from build123d import *

# Parameters (mm, degrees)
F0_R     = 8
F1_DEPTH = 16
F2_R     = 5.1
F3_DEPTH = 14
F4_R     = 5


with BuildPart() as f1:
    # F0 (on Top) → F1 (new body)
    with BuildSketch(Plane.XY):
        Circle(F0_R)
    extrude(amount=F1_DEPTH)

    # F2 (on face) → F3 (cut)
    with BuildSketch(Plane.XY.offset(16)):
        Circle(F2_R)
    extrude(amount=-F3_DEPTH, mode=Mode.SUBTRACT)

    # F4
    f4_edges = [f1.edges().sort_by_distance(p)[0] for p in [
        (-8, 0, 0),
    ]]
    fillet(f4_edges, radius=F4_R)


solid = f1.part
The listing builds one solid part. Answer for the finished solid, in the listing's coordinates (mm). A direction names the side the tool comes from. Round coordinates to 2 decimals unless told otherwise and drop trailing zeros. Order: outer loops, then holes, each group sorted by start corner. A loop starts at its lowest first (then second) coordinate and runs counter-clockwise, first axis right, second up. Notation, with made-up numbers: (-29.5, 83) -> (11.5, 83) arc R24 ccw to (11.5, 104) -> close; hole circle Ø1 at (0, -30.5). An arc over 180 degrees is marked (long way). Put each result on its own line as item: value.
Q1. Which of the six approach directions +Z, -Z, +X, -X, +Y, -Y give full straight-line access (tool end or side, diameter ignored) to faces 1 (the flat face through (0, 0, 0)), 2 (the flat face through (0, 0, 2))?
Results list:
face 1: -Z, +X, -X, +Y, -Y
face 2: +Z
Q2. Each of these flat-tipped pins is pushed along its axis until it touches: P1, Ø1.5, axis at x = -1, y = 1, coming from the -Z side; P2, Ø1, axis at y = -0.5, z = 2.5, coming from the -X side; P3, Ø1.5, axis at x = 3.5, z = 6.5, coming from the +Y side; P4, Ø4, axis at y = 4, z = 7.5, coming from the -X side. Where does it stop, or does it pass through?
Results list:
P1: z = 0
P2: x = -7.57
P3: y = 7.51
P4: x = -7.75
Q3. Determine the mould class of faces 3 (the flat face through (5, -2, 16)), 4 (the cylindrical face through (-1.73, -7.81, 10.42)), 5 (the cylindrical face through (2.4, -4.5, 9.1)) for opening direction Y: pulls with the +Y half, pulls with the -Y half, needs draft (parallel to the pull), parting line crosses it, or undercut.
Results list:
face 3: needs draft
face 4: parting line crosses it
face 5: undercut
Q4. Consider line 1 along Y through (x, z) = (0, 13); line 2 along X through (y, z) = (-4, 8); line 3 along Y through (x, z) = (-4.25, 7). Determine where each line is inside the solid, lowest interval first.
Results list:
line 1: -8 to -5.1, 5.1 to 8
line 2: -6.93 to -3.16, 3.16 to 6.93
line 3: -6.78 to -2.82, 2.82 to 6.78
Q5. Section A-A, the plane z = 11.25 is taken. Write down the section's boundary in (x, y), and give its area (3 significant figures).
Results list:
outline: circle Ø16 at (0, 0); hole circle Ø10.2 at (0, 0)
area: 119 mm^2
